```python
from build123d import *

# Parameters (mm, degrees)
BOSS_EXTRU_1_DEPTH = 5


with BuildPart() as part:
    # Esquisse1 → Boss.-Extru.1 (new body)
    with BuildSketch(Plane.XY):
        with BuildLine():
            Line((-10, 25), (-25, 25))
            Line((-25, 25), (-25, 10))
            Line((-25, 10), (-30, 10))
            Line((-30, 10), (-37, 10))
            Line((-37, 10), (-37, 5))
            Line((-37, 5), (-35, 5))
            Line((-35, 5), (-35, 6.5))
            Line((-35, 6.5), (-30, 6.5))
            Line((-30, 6.5), (-30, 5))
            Line((-30, 5), (-25, 5))
            Line((-25, 5), (-25, 0))
            Line((-25, 0), (-25, -5))
            Line((-25, -5), (-30, -5))
            Line((-30, -5), (-30, -6.5))
            Line((-30, -6.5), (-35, -6.5))
            Line((-35, -6.5), (-35, -5))
            Line((-35, -5), (-37, -5))
            Line((-37, -5), (-37, -10))
            Line((-37, -10), (-30, -10))
            Line((-30, -10), (-25, -10))
            Line((-25, -10), (-25, -25))
            Line((-25, -25), (-10, -25))
            Line((-10, -25), (-10, -30))
            Line((-10, -30), (-10, -37))
            Line((-10, -37), (-5, -37))
            Line((-5, -37), (-5, -35))
            Line((-5, -35), (-6.5, -35))
            Line((-6.5, -35), (-6.5, -30))
            Line((-6.5, -30), (-5, -30))
            Line((-5, -30), (-5, -25))
            Line((-5, -25), (-3.5, -25))
            Line((-3.5, -25), (-3.5, 0))
            ThreePointArc((-3.5, 0), (0, 3.5), (3.5, 0))
            Line((3.5, 0), (3.5, -25))
            Line((3.5, -25), (5, -25))
            Line((5, -25), (5, -30))
            Line((5, -30), (6.5, -30))
            Line((6.5, -30), (6.5, -35))
            Line((6.5, -35), (5, -35))
            Line((5, -35), (5, -37))
            Line((5, -37), (10, -37))
            Line((10, -37), (10, -30))
            Line((10, -30), (10, -25))
            Line((10, -25), (25, -25))
            Line((25, -25), (25, -10))
            Line((25, -10), (30, -10))
            Line((30, -10), (37, -10))
            Line((37, -10), (37, -5))
            Line((37, -5), (35, -5))
            Line((35, -5), (35, -6.5))
            Line((35, -6.5), (30, -6.5))
            Line((30, -6.5), (30, -5))
            Line((30, -5), (25, -5))
            Line((25, -5), (25, 0))
            Line((25, 0), (25, 5))
            Line((25, 5), (30, 5))
            Line((30, 5), (30, 6.5))
            Line((30, 6.5), (35, 6.5))
            Line((35, 6.5), (35, 5))
            Line((35, 5), (37, 5))
            Line((37, 5), (37, 10))
            Line((37, 10), (30, 10))
            Line((30, 10), (25, 10))
            Line((25, 10), (25, 25))
            Line((25, 25), (10, 25))
            Line((10, 25), (10, 30))
            Line((10, 30), (10, 37))
            Line((10, 37), (5, 37))
            Line((5, 37), (5, 35))
            Line((5, 35), (6.5, 35))
            Line((6.5, 35), (6.5, 30))
            Line((6.5, 30), (5, 30))
            Line((5, 30), (5, 25))
            Line((5, 25), (0, 25))
            Line((0, 25), (-5, 25))
            Line((-5, 25), (-5, 30))
            Line((-5, 30), (-6.5, 30))
            Line((-6.5, 30), (-6.5, 35))
            Line((-6.5, 35), (-5, 35))
            Line((-5, 35), (-5, 37))
            Line((-5, 37), (-10, 37))
            Line((-10, 37), (-10, 30))
            Line((-10, 30), (-10, 25))
        make_face()
    extrude(amount=BOSS_EXTRU_1_DEPTH)


solid = part.part
```
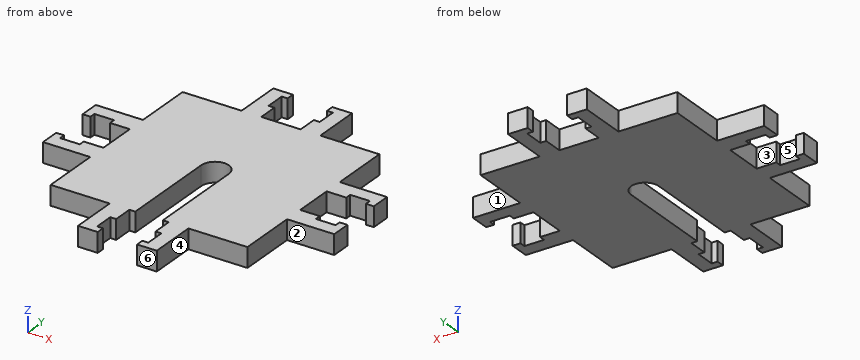
For this review, take the finished solid that the model builds, in its own axes (mm). Face numbers are marked on the shaded views. A direction names the side the tool comes from. Coordinates: 2 decimals unless noted, no trailing zeros. Order: outer loops, then holes, each group sorted by start corner. A loop starts at its lowest first (then second) coordinate and runs counter-clockwise, first axis right, second up. Notation, with made-up numbers: (50.25, 24.5) -> (74.25, 24.5) arc R26 cw to (74.25, 56.5) -> close; hole circle Ø2 at (6, 50). An arc over 180 degrees is marked (long way). Answer as CSV lines item,"result".
Q1. We need section B-B (x = 0). State the section outline as (y, z) points, plus the area to 4 significant figures.
Model answer:
outline,"(3.5, 0) -> (25, 0) -> (25, 5) -> (3.5, 5) -> close"
area,"107.5 mm2"
Q2. Clearance check with flat-ended pins moving along their axes: pin 1 Ø2.5 at (y, z) = (15, 1.5) entering from +X; pin 2 Ø2.5 at (x, z) = (20, 2.5) entering from -Y; pin 3 Ø2.5 at (x, z) = (27, 3.5) entering from +Y. State where each tip first meets the part, or that it passes through.
Model answer:
pin 1,"stops at x = 25"
pin 2,"stops at y = -25"
pin 3,"stops at y = 10"
Q3. For the marked faces 1, 2 and 3, list the 3-axis set-ups (+Z, -Z, +X, -X, +Y, -Y) from which the entire face can be reached by the end or side of a thin tool; tool diameter is ignored.
Model answer:
face 1,"+Z, -Z, +X, +Y"
face 2,"+Z, -Z, +X, -Y"
face 3,"+Z, -Z, -X"
Q4. We need section C-C (y = 16). State the section outline as (x, z) points, plus the area to 3 significant figures.
Model answer:
outline,"(-25, 0) -> (25, 0) -> (25, 5) -> (-25, 5) -> close"
area,"250 mm2"
Q5. Draft analysis for pull direction X (two halves, no side actions). For the marked faces 4, 5 and 6, state which applies: released by +X, released by -X, zero draft, split by the parting line, or undercut.
Model answer:
face 4,"released by +X"
face 5,"undercut"
face 6,"zero draft"
Q6. Wall thickness on line 1 along X through (y, z) = (-6, 3.6); line 2 along Y through (x, z) = (28, 3.8); line 3 along X through (y, z) = (34.5, 4): over which ranges is each line inside the solid? List them lowest first. Write a range as [from, to].
Model answer:
line 1,"x = [-37, -35], [-30, -3.5], [3.5, 30], [35, 37]"
line 2,"y = [-10, -5], [5, 10]"
line 3,"x = [-10, -6.5], [6.5, 10]"
Q7. We need section A-A (y = -16.5). State the section outline as (x, z) points.
Model answer:
outline,"(-25, 0) -> (-3.5, 0) -> (-3.5, 5) -> (-25, 5) -> close; (3.5, 0) -> (25, 0) -> (25, 5) -> (3.5, 5) -> close"
